```python
from build123d import *

# Parameters (mm, degrees)
ESQUISSE1_W        = 105.5
ESQUISSE1_H        = 75
ESQUISSE1_R        = 2
BOSS_EXTRU_1_DEPTH = 1.6
BOSS_EXTRU_2_DEPTH = 11
ESQUISSE6_W        = 13.2
ESQUISSE6_H        = 8
BOSS_EXTRU_3_DEPTH = 16
ESQUISSE7_W        = 71
ESQUISSE7_H        = 3.85
BOSS_EXTRU_4_DEPTH = 6.15
ESQUISSE8_W        = 48
ESQUISSE8_H        = 2.5
ESQUISSE8_W_2      = 39
ESQUISSE8_H_2      = 3.38327079
BOSS_EXTRU_5_DEPTH = 8.8
ESQUISSE9_W        = 5.75
ESQUISSE9_H        = 7.75
BOSS_EXTRU_6_DEPTH = 3


with BuildPart() as part:
    # Esquisse1 → Boss.-Extru.1 (new body)
    with BuildSketch(Plane.XY):
        Rectangle(ESQUISSE1_W, ESQUISSE1_H)
        with Locations((-48, 33)):
            Circle(ESQUISSE1_R, mode=Mode.SUBTRACT)
        with Locations((48, 33)):
            Circle(ESQUISSE1_R, mode=Mode.SUBTRACT)
        with Locations((-48, -33)):
            Circle(ESQUISSE1_R, mode=Mode.SUBTRACT)
        with Locations((48, -33)):
            Circle(ESQUISSE1_R, mode=Mode.SUBTRACT)
    extrude(amount=BOSS_EXTRU_1_DEPTH)

    # Esquisse5 → Boss.-Extru.2 (add)
    with BuildSketch(Plane(origin=(0, 0, 0), x_dir=(-1, 0, 0), z_dir=(0, 0, -1))):
        Polygon((-52.75, 30.2), (-31.75, 30.2), (-31.75, -29.5), (-55.75, -29.5), (-55.75, -20.5), (-52.75, -20.5), (-52.75, -6.5), (-56.5, -6.5), (-56.5, 0), (-52.75, 0), align=None)
    extrude(amount=BOSS_EXTRU_2_DEPTH)

    # Esquisse6 → Boss.-Extru.3 (add)
    with BuildSketch(Plane(origin=(0, 0, 0), x_dir=(-1, 0, 0), z_dir=(0, 0, -1))):
        with Locations((-36.15, -33.5)):
            Rectangle(ESQUISSE6_W, ESQUISSE6_H)
    extrude(amount=BOSS_EXTRU_3_DEPTH)

    # Esquisse7 → Boss.-Extru.4 (add)
    with BuildSketch(Plane(origin=(0, 0, 0), x_dir=(-1, 0, 0), z_dir=(0, 0, -1))):
        with Locations((8.55, -35.575)):
            Rectangle(ESQUISSE7_W, ESQUISSE7_H)
    extrude(amount=BOSS_EXTRU_4_DEPTH)

    # Esquisse8 → Boss.-Extru.5 (add)
    with BuildSketch(Plane(origin=(0, 0, 0), x_dir=(-1, 0, 0), z_dir=(0, 0, -1))):
        with Locations((11.55, 22.42)):
            Rectangle(ESQUISSE8_W, ESQUISSE8_H)
        with Locations((16.05, -26.308364605)):
            Rectangle(ESQUISSE8_W_2, ESQUISSE8_H_2)
    extrude(amount=BOSS_EXTRU_5_DEPTH)

    # Esquisse9 → Boss.-Extru.6 (add)
    with BuildSketch(Plane(origin=(0, 0, 0), x_dir=(-1, 0, 0), z_dir=(0, 0, -1))):
        with Locations((50.875, -1.625)):
            Rectangle(ESQUISSE9_W, ESQUISSE9_H)
    extrude(amount=BOSS_EXTRU_6_DEPTH)


solid = part.part
```
Check sheet for the modelled part. Datum: model origin and axes. Units: mm. A direction names the side the tool comes from. Round coordinates to 2 decimals unless told otherwise and drop trailing zeros. Order: outer loops, then holes, each group sorted by start corner. A loop starts at its lowest first (then second) coordinate and runs counter-clockwise, first axis right, second up. Notation, with made-up numbers: (12.5, 22.25) -> (63.5, 22.25) arc R17 ccw to (63.5, 54.25) -> close; hole circle Ø10 at (79, 75.25). An arc over 180 degrees is marked (long way). One line per item, written item: value. Start each with the question number.
Q1. Cross-section at C-C (x = 0). Record the boundary of the cut face in (y, z).
Q2. Gauge pin test, flat ends, axial feed: pin 1 Ø1 at (y, z) = (2.5, -4) entering from -X; pin 2 Ø1.1 at (x, z) = (54, -7.5) entering from -Y; pin 3 Ø1 at (x, z) = (-15, -10.5) entering from +Y; pin 4 Ø3.5 at (x, y) = (-8, -26.5) entering from -Z. Record the tip position at first contact, or that the pin passes through.
Q3. Set-up check for faces 1 (the face through (31.75, 1, -5)), 2 (the face through (42, 30.2, -5)), 3 (the face through (26.95, -36, -3)), 4 (the face through (-35.55, 22, -4)): record each of +Z, -Z, +X, -X, +Y, -Y from which the full face is reachable in a straight line by a thin tool's end or side.
Q4. Cross-section at D-D (y = -1.5). Record the boundary of the cut face in (x, z).
Q5. Thickness scan on line 1 (Y direction, x = -48, z = 0.6); line 2 (Y direction, x = 40, z = -8); line 3 (Z direction, x = 1, y = -18.5). Record the ranges inside material, lowest first.
Q6. Cross-section at B-B (y = 33). Record the boundary of the cut face in (x, z), and give its area (3 significant figures).
Q7. Mould release check, pull along X, two halves, no side actions. Record for faces 5 (the face through (56.5, -3, -5)), 6 (the face through (48, -35, 1)), 7 (the face through (-11, 22, -8.8)): pulls with the +X half, pulls with the -X half, needs draft (parallel to the pull), parting line crosses it, or undercut.
Q8. Cross-section at A-A (x = 48). Record the boundary of the cut face in (y, z), and give its area (3 significant figures).
Completed:
1. outline: (-37.5, -6.15) -> (-33.65, -6.15) -> (-33.65, 0) -> (-28, 0) -> (-28, -8.8) -> (-24.62, -8.8) -> (-24.62, 0) -> (21.17, 0) -> (21.17, -8.8) -> (23.67, -8.8) -> (23.67, 0) -> (37.5, 0) -> (37.5, 1.6) -> (-37.5, 1.6) -> close
2. pin 1: stops at x = 31.75
2. pin 2: stops at y = -29.5
2. pin 3: passes through
2. pin 4: stops at z = -8.8
3. face 1: -Z, +Y
3. face 2: -Z, +X, -X, +Y
3. face 3: -Z, +Y, -Y
3. face 4: -Z, -X, +Y
4. outline: (-53.75, -3) -> (-48, -3) -> (-48, 0) -> (31.75, 0) -> (31.75, -11) -> (56.5, -11) -> (56.5, 0) -> (52.75, 0) -> (52.75, 1.6) -> (-52.75, 1.6) -> (-52.75, 0) -> (-53.75, 0) -> close
5. line 1: y = -37.5 to -35, -31 to 31, 35 to 37.5
5. line 2: y = -37.5 to 30.2
5. line 3: z = 0 to 1.6
6. outline: (-52.75, 0) -> (-50, 0) -> (-50, 1.6) -> (-52.75, 1.6) -> close; (-46, 0) -> (46, 0) -> (46, 1.6) -> (-46, 1.6) -> close; (50, 0) -> (52.75, 0) -> (52.75, 1.6) -> (50, 1.6) -> close
6. area: 156 mm²
7. face 5: pulls with the +X half
7. face 6: undercut
7. face 7: needs draft
8. outline: (-37.5, 0) -> (-35, 0) -> (-35, 1.6) -> (-37.5, 1.6) -> close; (-31, 0) -> (-29.5, 0) -> (-29.5, -11) -> (30.2, -11) -> (30.2, 0) -> (31, 0) -> (31, 1.6) -> (-31, 1.6) -> close; (35, 0) -> (37.5, 0) -> (37.5, 1.6) -> (35, 1.6) -> close
8. area: 764 mm²
